Input: part model. Units: mm. Frame: model coordinates. A direction names the side the tool comes from. Coordinates: 2 decimals unless noted, no trailing zeros. Write each loop counter-clockwise with the first axis right and the second up, starting at its lowest first coordinate (ties: lowest second). Pieces come first, ordered by that corner, then holes. Notation, with made-up numbers: (-4.5, 55) - (17.5, 55) arc R29 cw to (17.5, 92) - close; hole circle Ø8 at (-16.5, 58). An arc over 180 degrees is marked (long way). Put each result on its own line as item: value. Start each with the question number.
1. Access query for faces 1 (the flat face through (-1, 27, 100)), 2 (the flat face through (64, 27, 1)). Directions: +Z, -Z, +X, -X, +Y, -Y. A direction counts if a zero-diameter tool reaches every point of the face in a straight line with its end or side. Return the directions, or none.
2. Line query: line 1 (X direction, y = 35.5, z = -51); line 2 (Z direction, x = 38, y = 24.5). Output: solid intervals per line, ascending.
3. Cut plane C-C, the plane y = 47.5. Return loops of the section in (x, z), and give its area (3 significant figures).
4. Pull-direction query (Z, two-part tool) for faces 3 (the cylindrical face through (-70.783, 27.115, -91.695)), 4 (the flat face through (-75, 27, -1)), 5 (the flat face through (1, 27, -100)); classes: released by +Z, released by -Z, zero draft, split by the parting line, or undercut.
5. Pin query (flat end, axial travel): pin 1 (9.5 mm diameter, centred on x = 69.32, z = 94.45, fed in from +Y); pin 2 (3.5 mm diameter, centred on x = -69.4, z = 94.37, fed in from -Y). Return the tip coordinate at first contact, or that it passes through.
6. Cut plane B-B, the plane x = 37.5. Return loops of the section in (y, z), and give its area (3 significant figures).
7. Cut plane A-A, the plane z = -80. Return loops of the section in (x, y), and give its area (3 significant figures).
Autodesk Inventor part; units mm, degrees
ref_plane "YZ Plane" through (0, 0, 0) normal (1, 0, 0) x (0, 1, 0)
ref_plane "XZ Plane" through (0, 0, 0) normal (0, 1, 0) x (-1, 0, 0)
ref_plane "XY Plane" through (0, 0, 0) normal (0, 0, 1) x (1, 0, 0)
sketch "Sketch1" plane through (0, 0, 0) normal (0, 1, 0) x (-1, 0, 0)
  line L0 (-75, 0) -> (-75, -100)
  line L1 (-75, -100) -> (75, -100)
  line L2 (75, -100) -> (75, 100)
  line L3 (75, 100) -> (-75, 100)
  line L4 (-75, 100) -> (-75, 0)
  circle A0 centre (69.3987, -94.3567) radius 3
  circle A1 centre (-69.3245, -94.3567) radius 3
  circle A2 centre (69.3987, 94.3688) radius 3
  circle A3 centre (-69.3245, 94.4539) radius 3
  line L5 (75, -100) -> (75, -97.4)
  line L6 (75, 100) -> (57, 100)
  line L7 (75, 100) -> (64, 100)
  line L8 (64, 100) -> (64, -100)
  line L9 (-75, 100) -> (-64, 100)
  line L10 (-64, 100) -> (-64, -100)
  line L11 (64, -100) -> (64, -89)
  line L12 (64, -89) -> (-64, -89)
  line L13 (64, 100) -> (64, 89)
  line L14 (64, 89) -> (-64, 89)
  point P0 (0, 0)
  dimension "d3" = 200
  dimension "d4" = 150
  dimension "d5" = 6
  dimension "d6" = 6
  dimension "d7" = 6
  dimension "d8" = 6
  dimension "d18" = 11
extrude "Extrusion1" add sketch "Sketch1" along normal blind 55 contours L3 L8 L14 L10
extrude "Extrusion2" add sketch "Sketch1" along normal blind 55 contours L8 L3 L2 L1
extrude "Extrusion3" add sketch "Sketch1" along normal blind 55 contours L4 L3 L10 L1 L0
extrude "Extrusion4" add sketch "Sketch1" along normal blind 55 contours L10 L12 L8 L1
Report:
1. face 1: +Z, +X, -X, +Y, -Y
1. face 2: +Y, -Y
2. line 1: x = -75 to -64, 64 to 75
2. line 2: z = -100 to -89, 89 to 100
3. outline: (-75, -100) - (75, -100) - (75, 100) - (-75, 100) - close; hole circle Ø6 at (-69.4, -94.36); hole circle Ø6 at (-69.4, 94.37); hole (-64, -89) - (64, -89) - (64, 89) - (-64, 89) - close; hole circle Ø6 at (69.32, -94.36); hole circle Ø6 at (69.32, 94.45)
3. area: 7,100 mm^2
4. face 3: undercut
4. face 4: zero draft
4. face 5: released by -Z
5. pin 1: stops at y = 55
5. pin 2: passes through
6. outline: (0, -100) - (55, -100) - (55, -89) - (0, -89) - close; (0, 89) - (55, 89) - (55, 100) - (0, 100) - close
6. area: 1,210 mm^2
7. outline: (-75, 0) - (-64, 0) - (-64, 55) - (-75, 55) - close; (64, 0) - (75, 0) - (75, 55) - (64, 55) - close
7. area: 1,210 mm^2
